```python
from build123d import *

# Parameters (mm, degrees)
F1_DEPTH = 6.35


with BuildPart() as f1:
    # F0 (on Right) → F1 (new body)
    with BuildSketch(Plane.YZ):
        with BuildLine():
            ThreePointArc((-141.971718, 29.874661), (-143.09425, 30.339629), (-143.559218, 31.462161))
            Line((-143.559218, 31.462161), (-148.321718, 31.462161))
            Line((-148.321718, 31.462161), (-148.321718, 12.412161))
            Line((-148.321718, 12.412161), (-143.559218, 12.412161))
            ThreePointArc((-143.559218, 12.412161), (-143.09425, 13.534693), (-141.971718, 13.999661))
            Line((-141.971718, 13.999661), (-141.971718, 29.874661))
        make_face()
        with BuildLine():
            Line((156.478282, 50.512161), (-141.971718, 50.512161))
            Line((-141.971718, 50.512161), (-141.971718, 33.049661))
            ThreePointArc((-141.971718, 33.049661), (-140.849186, 32.584693), (-140.384218, 31.462161))
            ThreePointArc((-140.384218, 31.462161), (-140.849186, 30.339629), (-141.971718, 29.874661))
            Line((-141.971718, 29.874661), (-141.971718, 13.999661))
            ThreePointArc((-141.971718, 13.999661), (-140.849186, 13.534693), (-140.384218, 12.412161))
            ThreePointArc((-140.384218, 12.412161), (-140.849186, 11.289629), (-141.971718, 10.824661))
            Line((-141.971718, 10.824661), (-141.971718, -0.287839))
            Line((-141.971718, -0.287839), (-105.459218, -0.287839))
            ThreePointArc((-105.459218, -0.287839), (-103.871718, 1.299661), (-102.284218, -0.287839))
            Line((-102.284218, -0.287839), (-86.409218, -0.287839))
            ThreePointArc((-86.409218, -0.287839), (-84.821718, 1.299661), (-83.234218, -0.287839))
            Line((-83.234218, -0.287839), (-3.859218, -0.287839))
            ThreePointArc((-3.859218, -0.287839), (-2.271718, 1.299661), (-0.684218, -0.287839))
            Line((-0.684218, -0.287839), (15.190782, -0.287839))
            ThreePointArc((15.190782, -0.287839), (16.778282, 1.299661), (18.365782, -0.287839))
            Line((18.365782, -0.287839), (97.740782, -0.287839))
            ThreePointArc((97.740782, -0.287839), (99.328282, 1.299661), (100.915782, -0.287839))
            Line((100.915782, -0.287839), (116.790782, -0.287839))
            ThreePointArc((116.790782, -0.287839), (118.378282, 1.299661), (119.965782, -0.287839))
            Line((119.965782, -0.287839), (156.478282, -0.287839))
            Line((156.478282, -0.287839), (156.478282, 10.824661))
            ThreePointArc((156.478282, 10.824661), (154.890782, 12.412161), (156.478282, 13.999661))
            Line((156.478282, 13.999661), (156.478282, 29.874661))
            ThreePointArc((156.478282, 29.874661), (154.890782, 31.462161), (156.478282, 33.049661))
            Line((156.478282, 33.049661), (156.478282, 50.512161))
        make_face()
        with BuildLine():
            ThreePointArc((-46.721718, 29.874661), (-47.84425, 32.584693), (-45.134218, 31.462161))
            Line((-45.134218, 31.462161), (-41.959218, 31.462161))
            ThreePointArc((-41.959218, 31.462161), (-40.371718, 33.049661), (-38.784218, 31.462161))
            ThreePointArc((-38.784218, 31.462161), (-39.249186, 30.339629), (-40.371718, 29.874661))
            Line((-40.371718, 29.874661), (-40.371718, 13.999661))
            ThreePointArc((-40.371718, 13.999661), (-39.249186, 13.534693), (-38.784218, 12.412161))
            ThreePointArc((-38.784218, 12.412161), (-40.371718, 10.824661), (-41.959218, 12.412161))
            Line((-41.959218, 12.412161), (-45.134218, 12.412161))
            ThreePointArc((-45.134218, 12.412161), (-47.84425, 11.289629), (-46.721718, 13.999661))
            Line((-46.721718, 13.999661), (-46.721718, 29.874661))
        make_face(mode=Mode.SUBTRACT)
        with BuildLine():
            ThreePointArc((54.878282, 29.874661), (53.75575, 32.584693), (56.465782, 31.462161))
            Line((56.465782, 31.462161), (59.640782, 31.462161))
            ThreePointArc((59.640782, 31.462161), (61.228282, 33.049661), (62.815782, 31.462161))
            ThreePointArc((62.815782, 31.462161), (62.350814, 30.339629), (61.228282, 29.874661))
            Line((61.228282, 29.874661), (61.228282, 13.999661))
            ThreePointArc((61.228282, 13.999661), (62.350814, 13.534693), (62.815782, 12.412161))
            ThreePointArc((62.815782, 12.412161), (61.228282, 10.824661), (59.640782, 12.412161))
            Line((59.640782, 12.412161), (56.465782, 12.412161))
            ThreePointArc((56.465782, 12.412161), (53.75575, 11.289629), (54.878282, 13.999661))
            Line((54.878282, 13.999661), (54.878282, 29.874661))
        make_face(mode=Mode.SUBTRACT)
        with BuildLine():
            Line((-86.409218, -0.287839), (-102.284218, -0.287839))
            ThreePointArc((-102.284218, -0.287839), (-102.749186, -1.410371), (-103.871718, -1.875339))
            Line((-103.871718, -1.875339), (-103.871718, -6.637839))
            Line((-103.871718, -6.637839), (-84.821718, -6.637839))
            Line((-84.821718, -6.637839), (-84.821718, -1.875339))
            ThreePointArc((-84.821718, -1.875339), (-85.94425, -1.410371), (-86.409218, -0.287839))
        make_face()
        with BuildLine():
            ThreePointArc((16.778282, -1.875339), (15.65575, -1.410371), (15.190782, -0.287839))
            Line((15.190782, -0.287839), (-0.684218, -0.287839))
            ThreePointArc((-0.684218, -0.287839), (-1.149186, -1.410371), (-2.271718, -1.875339))
            Line((-2.271718, -1.875339), (-2.271718, -6.637839))
            Line((-2.271718, -6.637839), (16.778282, -6.637839))
            Line((16.778282, -6.637839), (16.778282, -1.875339))
        make_face()
        with BuildLine():
            ThreePointArc((118.378282, -1.875339), (117.25575, -1.410371), (116.790782, -0.287839))
            Line((116.790782, -0.287839), (100.915782, -0.287839))
            ThreePointArc((100.915782, -0.287839), (100.450814, -1.410371), (99.328282, -1.875339))
            Line((99.328282, -1.875339), (99.328282, -6.637839))
            Line((99.328282, -6.637839), (118.378282, -6.637839))
            Line((118.378282, -6.637839), (118.378282, -1.875339))
        make_face()
        with BuildLine():
            Line((162.828282, 31.462161), (158.065782, 31.462161))
            ThreePointArc((158.065782, 31.462161), (157.600814, 30.339629), (156.478282, 29.874661))
            Line((156.478282, 29.874661), (156.478282, 13.999661))
            ThreePointArc((156.478282, 13.999661), (157.600814, 13.534693), (158.065782, 12.412161))
            Line((158.065782, 12.412161), (162.828282, 12.412161))
            Line((162.828282, 12.412161), (162.828282, 31.462161))
        make_face()
    extrude(amount=F1_DEPTH)


solid = f1.part
```
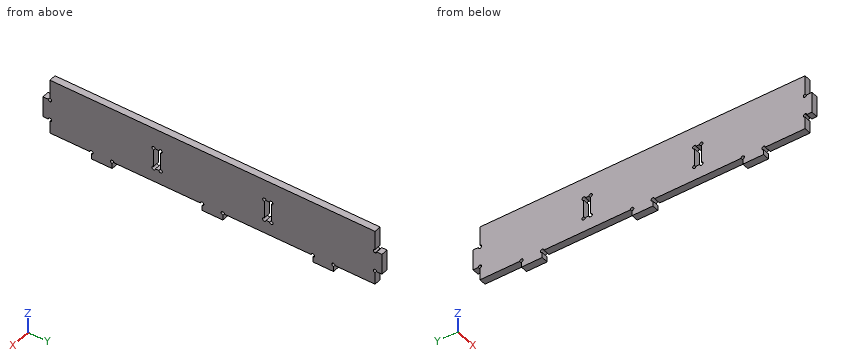
The listing builds one solid part. Answer for the finished solid, in the listing's coordinates (mm). Give positions to 0.01 mm unless a question says otherwise; leave off trailing zeros. Order: outer loops, then holes, each group sorted by start corner. A loop starts at its lowest first (then second) coordinate and runs counter-clockwise, first axis right, second up. Notation, with made-up numbers: (70.25, 32.5) - (93.25, 32.5) arc R21 ccw to (93.25, 57.5) - close; hole circle Ø4 at (39.25, -7.75). An arc over 180 degrees is marked (long way). Use one line per item in the form item = value. Start each with the question number.
(1) A cutting plane is placed at C-C, the plane x = 4.5. State how many separate pieces and enclosed holes the cut face has, then the cut area to 3 significant figures.
(2) A cutting plane is placed at B-B, the plane y = -25. Write down the section's boundary in (x, z), then the cut area to 3 significant figures.
(3) A cutting plane is placed at D-D, the plane z = 37. Write down the section's boundary in (x, y), then the cut area to 3 significant figures.
(4) Flat-ended cylindrical pins translate along their axes: pin 1 Ø1.4 at (x, z) = (2, -5.5) entering from +Y; pin 2 Ø2.5 at (x, z) = (2.5, -5.5) entering from -Y. Find the tip coordinate at first contact, or state that the pin passes through.
(5) Consider line 1 (Y direction, x = 6, z = 25); line 2 (Y direction, x = 3.5, z = -2); line 3 (Y direction, x = 5, z = 8). Determine where each line is inside the solid, lowest interval first. Write a range as from..to.
(6) A cutting plane is placed at A-A, the plane z = 17. Write down the section's boundary in (x, y).
Ans:
q1.separate_pieces = 1
q1.enclosed_holes = 2
q1.area = 15,400 mm^2
q2.outline = (0, -0.29) - (6.35, -0.29) - (6.35, 50.51) - (0, 50.51) - close
q2.area = 323 mm^2
q3.outline = (0, -141.97) - (6.35, -141.97) - (6.35, 156.48) - (0, 156.48) - close
q3.area = 1,900 mm^2
q4.pin_1 = 118.38
q4.pin_2 = -103.87
q5.line_1 = -148.32..-46.72, -40.37..54.88, 61.23..162.83
q5.line_2 = -103.87..-84.82, -2.27..16.78, 99.33..118.38
q5.line_3 = -141.97..156.48
q6.outline = (0, -148.32) - (6.35, -148.32) - (6.35, -46.72) - (0, -46.72) - close; (0, -40.37) - (6.35, -40.37) - (6.35, 54.88) - (0, 54.88) - close; (0, 61.23) - (6.35, 61.23) - (6.35, 162.83) - (0, 162.83) - close
